Check sheet for the modelled part. Datum: model origin and axes. Units: mm. Face numbers are marked on the shaded views. Coordinates: 2 decimals unless noted, no trailing zeros. Loops run counter-clockwise (first coordinate to the right, second up) from the corner with the lowest first, then second, coordinate; pieces in that order, holes last. Notation, with made-up numbers: M 0.25,-15 L 58.25,-15 A30 ccw 58.25,21 Z; hole C 68.25,-10.75 d6. An arc over 180 degrees is marked long. Answer in a Markdown table with one row per item. Add a question column.
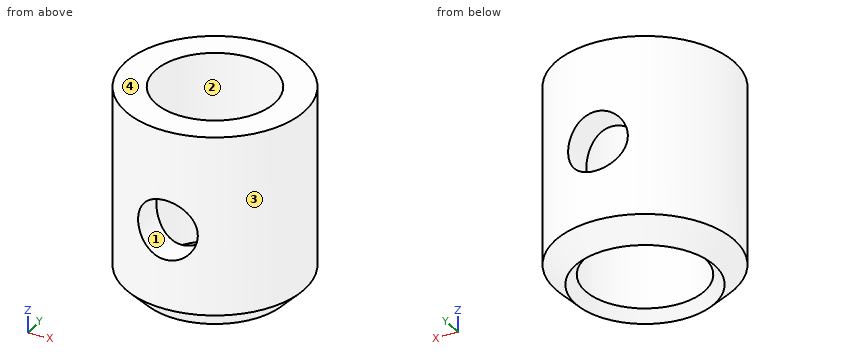
```python
from build123d import *

# Parameters (mm, degrees)
ESQUISSE1_R                  = 9
ESQUISSE1_R_2                = 6
BASE_EXTRUSION_DEPTH         = 20
CHANFREIN1_SIZE              = 2
ENL_V_MAT_EXTRU_1_DEPTH      = 20
ENL_V_MAT_EXTRU_1_DEPTH_BACK = 24.706539182
ESQUISSE2_R                  = 3
CHANFREIN2_SIZE              = 1


with BuildPart() as part:
    # Esquisse1 → Base-Extrusion (new body)
    with BuildSketch(Plane.XY):
        Circle(ESQUISSE1_R)
        Circle(ESQUISSE1_R_2, mode=Mode.SUBTRACT)
    extrude(amount=BASE_EXTRUSION_DEPTH)

    # Chanfrein1
    chanfrein1_edges = [part.edges().sort_by_distance(p)[0] for p in [
        (-9, 0, 0),
    ]]
    chamfer(chanfrein1_edges, length=CHANFREIN1_SIZE - 0.0001)  # a hair under: the kernel refuses the full size

    # Esquisse2 → Enlèv. mat.-Extru.1 (cut, two sides: drawn at the far end of the back side and taken through both)
    with BuildSketch(Plane(origin=(0, 0, 0), x_dir=(1, 0, 0), z_dir=(0, 1, 0)).offset(-ENL_V_MAT_EXTRU_1_DEPTH_BACK)):
        with Locations(Location((0, -10, 0), (0, 0, 270))):
            Circle(ESQUISSE2_R)
    extrude(amount=ENL_V_MAT_EXTRU_1_DEPTH + ENL_V_MAT_EXTRU_1_DEPTH_BACK, mode=Mode.SUBTRACT)

    # Chanfrein2
    chanfrein2_edges = [part.edges().sort_by_distance(p)[0] for p in [
        (-6, 0, 0),
    ]]
    chamfer(chanfrein2_edges, length=CHANFREIN2_SIZE)


solid = part.part
```
Q1. Thickness scan on L1, parallel to Y at x = 0, z = 16.25; L2, parallel to Y at x = -2.5, z = 4.25; L3, parallel to X at y = -2, z = 3.25. Record the ranges inside material, lowest first.
Q2. Cross-section at D-D (z = 18.5). Record the cut outline in (x, y).
Q3. Go/stop test with flat-tipped pins: pin 1 (1 mm diameter, centred on y = 2, z = 4, fed in from -X); pin 2 (3 mm diameter, centred on x = 0.5, y = -3.5, fed in from -Z); pin 3 (3 mm diameter, centred on x = 6.5, z = 4, fed in from -Y); pin 4 (5 mm diameter, centred on x = -7, z = 6.5, fed in from +Y). Record where each tip stops, or that it passes through.
Q4. Cross-section at C-C (z = 10). Record the cut outline in (x, y), plus the area to 3 significant figures.
Q5. Cross-section at B-B (x = 0). Count the separate pieces of the cut face and the enclosed holes in it, plus the area to 3 significant figures.
Q6. Mould release check, pull along X, two halves, no side actions. Record for the marked faces 1, 2, 3 and 4: released by +X, released by -X, zero draft, split by the parting line, or undercut.
Answer key:
| question | item | result |
|---|---|---|
| 1 | L1 | -9 to -6, 6 to 9 |
| 1 | L2 | -8.65 to -5.45, 5.45 to 8.65 |
| 1 | L3 | -8.77 to -5.66, 5.66 to 8.77 |
| 2 | outline | C 0,0 d18; hole C 0,0 d12 |
| 3 | pin 1 | x = -8.87 |
| 3 | pin 2 | through |
| 3 | pin 3 | y = -7.48 |
| 3 | pin 4 | y = 7.79 |
| 4 | outline | M -3,-8.49 L -3,-5.2 A6 cw -3,5.2 L -3,8.49 A9 ccw Z; M 3,-8.49 A9 ccw 3,8.49 L 3,5.2 A6 cw 3,-5.2 Z |
| 4 | area | 104 mm^2 |
| 5 | separate pieces | 4 |
| 5 | enclosed holes | 0 |
| 5 | area | 79.0 mm^2 |
| 6 | face 1 | undercut |
| 6 | face 2 | undercut |
| 6 | face 3 | split by the parting line |
| 6 | face 4 | zero draft |
